Model file for the job. Use its own axes, mm. Give positions to 0.01 mm unless a question says otherwise; leave off trailing zeros. Loops run counter-clockwise (first coordinate to the right, second up) from the corner with the lowest first, then second, coordinate; pieces in that order, holes last. Notation, with made-up numbers: (22, 21.5) -> (57, 21.5) arc R16 ccw to (57, 32.5) -> close; hole circle Ø5 at (-16.75, -37). An arc over 180 degrees is marked (long way). Use CSV: the item, a comma, the result in double quotes. Start each with the question number.
(1) Cut at C-C on z = 1.45. State how many separate pieces and enclosed holes the cut face has, then the cut area to 3 significant figures.
(2) Cut at A-A on y = 17.5. Write the cut outline in (x, z).
(3) Flat gauge pins, fed straight in: pin 1 (0.6 mm diameter, centred on x = 50.5, z = 1.5, fed in from -Y) (3 decimals); pin 2 (2 mm diameter, centred on x = 22.275, y = 21.065, fed in from +Z). Where does each tip first touch, or does it go through?
(4) Drill centre lines: probe 1 along X at (y, z) = (17, 1.65); probe 2 along X at (y, z) = (29.5, 1.3); probe 3 along Y at (x, z) = (51.5, 0.3) (3 decimals). Where is each one in solid material? Low to high.
(5) Cut at D-D on y = 27.75. Write the cut outline in (x, z), then the cut area to 3 significant figures.
(6) Cut at B-B on x = 56.5. Write the cut outline in (y, z) (3 decimals).
from build123d import *

# Parameters (mm, degrees)
BOSS_EXTRUDE1_DEPTH = 2.032
FILLET1_R           = 5
FILLET4_R           = 2
SKETCH5_R           = 1.190625
CUT_EXTRUDE1_DEPTH  = 75.011460165


with BuildPart() as part:
    # Sketch3 → Boss-Extrude1 (new body)
    with BuildSketch(Plane.XY):
        with BuildLine():
            Line((61.234837488, 27.025), (44.888079179, 27.025))
            Line((44.888079179, 27.025), (45.635822761, 28.585508346))
            ThreePointArc((45.635822761, 28.585508346), (42.595854881, 29.183740622), (40.224926589, 31.178229429))
            Line((40.224926589, 31.178229429), (38.234837488, 27.025))
            Line((38.234837488, 27.025), (21.888079179, 27.025))
            Line((21.888079179, 27.025), (22.635822761, 28.585508346))
            ThreePointArc((22.635822761, 28.585508346), (19.595854881, 29.183740622), (17.224926589, 31.178229429))
            Line((17.224926589, 31.178229429), (10.414177239, 16.964491654))
            ThreePointArc((10.414177239, 16.964491654), (13.454145119, 16.366259378), (15.825073411, 14.371770571))
            Line((15.825073411, 14.371770571), (17.815162512, 18.525))
            Line((17.815162512, 18.525), (34.161920821, 18.525))
            Line((34.161920821, 18.525), (33.414177239, 16.964491654))
            ThreePointArc((33.414177239, 16.964491654), (36.454145119, 16.366259378), (38.825073411, 14.371770571))
            Line((38.825073411, 14.371770571), (40.815162512, 18.525))
            Line((40.815162512, 18.525), (57.161920821, 18.525))
            Line((57.161920821, 18.525), (56.414177239, 16.964491654))
            ThreePointArc((56.414177239, 16.964491654), (59.454145119, 16.366259378), (61.825073411, 14.371770571))
            Line((61.825073411, 14.371770571), (68.635822761, 28.585508346))
            ThreePointArc((68.635822761, 28.585508346), (65.595854881, 29.183740622), (63.224926589, 31.178229429))
            Line((63.224926589, 31.178229429), (61.234837488, 27.025))
        make_face()
    extrude(amount=BOSS_EXTRUDE1_DEPTH)

    # Fillet1
    fillet1_edges = [part.edges().sort_by_distance(p)[0] for p in [
        (38.234837488, 27.025, 1.016),
        (61.234837488, 27.025, 1.016),
        (40.815162512, 18.525, 1.016),
        (17.815162512, 18.525, 1.016),
    ]]
    fillet(fillet1_edges, radius=FILLET1_R)

    # Fillet4
    # the kernel refuses this fillet: 2 mm, written as the material it takes off along each edge
    with BuildSketch(Plane(origin=(61.825073411, 14.371770571, -6.782329983), x_dir=(-0.7244869564055234, 0.6892885099856672, 0), z_dir=(0, 0, 1))) as fillet4_piece_1:
        with BuildLine():
            CenterArc((2.739483145, -1.963474497), FILLET4_R, 100.966900666, 97.004726409)
            Line((0.837064294, -2.580566482), (0.799015917, -2.592908322))
            Line((0.799015917, -2.592908322), (-0.038048377, -0.01234184))
            Line((-0.038048377, -0.01234184), (0.007609675, 0.03926949))
            ThreePointArc((0.007609675, 0.03926949), (1.179499687, -0.073229059), (2.351389699, 0.03926949))
            Line((2.351389699, 0.03926949), (2.358999374, 0))
        make_face()
    extrude(amount=15.596659966, mode=Mode.SUBTRACT)
    with BuildSketch(Plane(origin=(56.414177239, 16.964491654, -5.447751417), x_dir=(0.4321201804305817, 0.9018160287246183, 0), z_dir=(0, 0, 1)), Plane(origin=(33.414177239, 16.964491654, -5.447751417), x_dir=(0.4321201804305726, 0.9018160287246226, 0), z_dir=(0, 0, 1))) as fillet4_piece_2:
        with BuildLine():
            CenterArc((2.679877065, -1.760257284), FILLET4_R, 118.342114692, 70.353672363)
            Line((0.702867053, -2.062633556), (0.663326852, -2.068681081))
            ThreePointArc((0.663326852, -2.068681081), (0.404900733, -1.013097188), (-0.035005574, -0.019354839))
            Line((-0.035005574, -0.019354839), (0, 0.04))
            ThreePointArc((0, 0.04), (0.865203266, 0.04), (1.71141712, 0.035205146))
            Line((1.71141712, 0.035205146), (1.730406531, 0))
        make_face()
    extrude(amount=12.927502834, mode=Mode.SUBTRACT)
    with BuildSketch(Plane(origin=(68.635822761, 28.585508346, -6.782329983), x_dir=(-0.43212018043056016, -0.9018160287246285, 0), z_dir=(0, 0, 1))) as fillet4_piece_3:
        with BuildLine():
            CenterArc((2.712931993, -2), FILLET4_R, 90, 97.004726409)
            Line((0.727859803, -2.243902439), (0.688158359, -2.248780488))
            ThreePointArc((0.688158359, -2.248780488), (0.433586073, -1.099356687), (-0.035005574, -0.019354839))
            Line((-0.035005574, -0.019354839), (0, 0.04))
            Line((0, 0.04), (2.712931993, 0.04))
            Line((2.712931993, 0.04), (2.712931993, 0))
        make_face()
    extrude(amount=15.596659966, mode=Mode.SUBTRACT)
    with BuildSketch(Plane(origin=(63.224926589, 31.178229429, -5.862766834), x_dir=(0.7197655743666583, -0.6942171979695075, 0), z_dir=(0, 0, 1)), Plane(origin=(38.825073411, 14.371770571, -5.862766834), x_dir=(-0.7197655743666577, 0.6942171979695083, 0), z_dir=(0, 0, 1))) as fillet4_piece_4:
        with BuildLine():
            CenterArc((2.642931874, -1.966025629), FILLET4_R, 100.575844506, 87.569716535)
            Line((0.663109271, -2.249402518), (0.465127011, -2.277740206))
            ThreePointArc((0.465127011, -2.277740206), (0.269143449, -1.445696099), (-0.189816279, -0.063006193))
            Line((-0.189816279, -0.063006193), (0.036707387, 0.196602563))
            ThreePointArc((0.036707387, 0.196602563), (1.137929001, 0.094679449), (2.239150616, 0.196602563))
            Line((2.239150616, 0.196602563), (2.275858003, 0))
        make_face()
    extrude(amount=13.757533668, mode=Mode.SUBTRACT)
    with BuildSketch(Plane(origin=(45.635822761, 28.585508346, -5.447751417), x_dir=(-0.992996409987433, 0.11814452908226362, 0), z_dir=(0, 0, 1)), Plane(origin=(22.635822761, 28.585508346, -5.447751417), x_dir=(-0.9929964099874332, 0.11814452908226183, 0), z_dir=(0, 0, 1))) as fillet4_piece_5:
        with BuildLine():
            CenterArc((2.5305684, 1.968875405), FILLET4_R, 189.524957294, 70.353672363)
            Line((0.558141169, 1.637920999), (0.518692625, 1.631301911))
            ThreePointArc((0.518692625, 1.631301911), (0.241208476, 0.831862466), (-0.037862109, 0.012901966))
            Line((-0.037862109, 0.012901966), (0.007029357, -0.039377508))
            ThreePointArc((0.007029357, -0.039377508), (1.089550283, 0.056486243), (2.17207121, -0.039377508))
            Line((2.17207121, -0.039377508), (2.179100567, 0))
        make_face()
    extrude(amount=12.927502834, mode=Mode.SUBTRACT)
    with BuildSketch(Plane(origin=(40.224926589, 31.178229429, -5.862766834), x_dir=(-0.4623630437345738, -0.8866907103316808, 0), z_dir=(0, 0, 1)), Plane(origin=(15.825073411, 14.371770571, -5.862766834), x_dir=(0.46236304373457116, 0.886690710331682, 0), z_dir=(0, 0, 1))) as fillet4_piece_6:
        with BuildLine():
            CenterArc((2.633114962, 1.979154178), FILLET4_R, 174.150669546, 87.569716535)
            Line((0.643528297, 2.18297984), (0.44456963, 2.203362406))
            ThreePointArc((0.44456963, 2.203362406), (0.230948584, 1.118261759), (-0.178199689, 0.090801271))
            Line((-0.178199689, 0.090801271), (0.006761891, -0.199885659))
            ThreePointArc((0.006761891, -0.199885659), (1.462800781, -0.150629619), (2.316305911, -0.197915418))
            Line((2.316305911, -0.197915418), (2.345106734, 0))
        make_face()
    extrude(amount=13.757533668, mode=Mode.SUBTRACT)
    with BuildSketch(Plane(origin=(10.414177239, 16.964491654, -6.782329983), x_dir=(0.9911448562189062, -0.13278506689685937, 0), z_dir=(0, 0, 1))) as fillet4_piece_7:
        with BuildLine():
            CenterArc((2.739483145, 1.963474497), FILLET4_R, 162.028372925, 97.004726409)
            Line((0.837064294, 2.580566482), (0.799015917, 2.592908322))
            Line((0.799015917, 2.592908322), (-0.038048377, 0.01234184))
            Line((-0.038048377, 0.01234184), (0.007609675, -0.03926949))
            ThreePointArc((0.007609675, -0.03926949), (1.179499687, 0.073229059), (2.351389699, -0.03926949))
            Line((2.351389699, -0.03926949), (2.358999374, 0))
        make_face()
    extrude(amount=15.596659966, mode=Mode.SUBTRACT)
    with BuildSketch(Plane(origin=(17.224926589, 31.178229429, -6.782329983), x_dir=(-0.4321201804305535, -0.9018160287246317, 0), z_dir=(0, 0, 1))) as fillet4_piece_8:
        with BuildLine():
            CenterArc((2.712931993, 2), FILLET4_R, 172.995273591, 97.004726409)
            Line((0.727859803, 2.243902439), (0.688158359, 2.248780488))
            ThreePointArc((0.688158359, 2.248780488), (0.433586073, 1.099356687), (-0.035005574, 0.019354839))
            Line((-0.035005574, 0.019354839), (0, -0.04))
            Line((0, -0.04), (2.712931993, -0.04))
            Line((2.712931993, -0.04), (2.712931993, 0))
        make_face()
    extrude(amount=15.596659966, mode=Mode.SUBTRACT)

    # Sketch5 → Cut-Extrude1 (cut, through all)
    with BuildSketch(Plane.XY.offset(2.032)):
        with Locations((22.275, 21.065)):
            Circle(SKETCH5_R)
        with Locations((56.775, 24.485)):
            Circle(SKETCH5_R)
    extrude(amount=-CUT_EXTRUDE1_DEPTH, mode=Mode.SUBTRACT)


solid = part.part
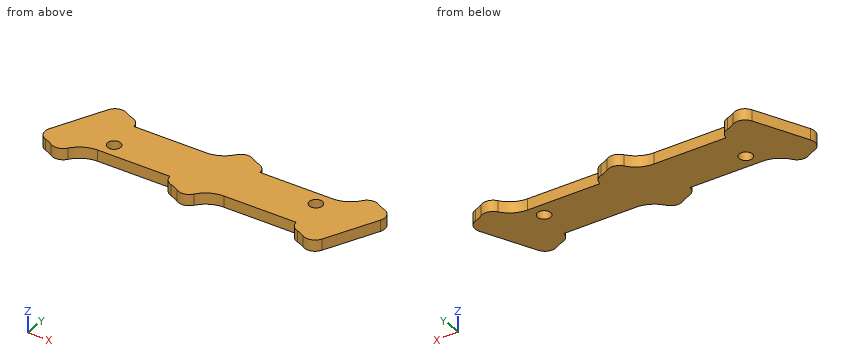
Check result:
1,separate pieces,"1"
1,enclosed holes,"2"
1,area,"525 mm²"
2,outline,"(11.69, 0) -> (17.93, 0) -> (17.93, 2.03) -> (11.69, 2.03) -> close; (34.5, 0) -> (40.93, 0) -> (40.93, 2.03) -> (34.5, 2.03) -> close; (57.5, 0) -> (63.32, 0) -> (63.32, 2.03) -> (57.5, 2.03) -> close"
3,pin 1,"y = 18.525"
3,pin 2,"through"
4,probe 1,"12.12 to 17.37, 34.99 to 40.37, 57.99 to 63.08"
4,probe 2,"16.7 to 19.02, 39.53 to 42.02, 62.53 to 65.02"
4,probe 3,"18.525 to 27.025"
5,outline,"(15.58, 0) -> (21.71, 0) -> (21.71, 2.03) -> (15.58, 2.03) -> close; (37.68, 0) -> (44.71, 0) -> (44.71, 2.03) -> (37.68, 2.03) -> close; (60.68, 0) -> (67.52, 0) -> (67.52, 2.03) -> (60.68, 2.03) -> close"
5,area,"40.6 mm²"
6,outline,"(18.525, 0) -> (23.327, 0) -> (23.327, 2.032) -> (18.525, 2.032) -> close; (25.643, 0) -> (27.025, 0) -> (27.025, 2.032) -> (25.643, 2.032) -> close"
